from build123d import *

# Parameters (mm, degrees)
CYLINDER018_R               = 0.6
CYLINDER018_DEPTH           = 30
CYLINDER018_PLACEMENT_ANGLE = 45
ARRAY_COUNT                 = 6
CYLINDER014_R               = 0.4
CYLINDER014_DEPTH           = 2
CYLINDER012_R               = 0.41
CYLINDER012_DEPTH           = 0.8
CYLINDER013_R               = 0.7
CYLINDER013_DEPTH           = 0.55
FILLET003_R                 = 0.24
CYLINDER015_R               = 5
CYLINDER015_DEPTH           = 0.1
CYLINDER008_R               = 16
CYLINDER008_DEPTH           = 10
CYLINDER007_R               = 14
CYLINDER007_DEPTH           = 6.4
CYLINDER006_R               = 14
CYLINDER006_DEPTH           = 1
CYLINDER005_R               = 0.4
CYLINDER005_DEPTH           = 1
CYLINDER001_R               = 12.6
CYLINDER001_DEPTH           = 8
CYLINDER_R                  = 15
CYLINDER_DEPTH              = 8
CYLINDER002_R               = 15
CYLINDER002_DEPTH           = 1
FILLET_R                    = 0.7
FILLET001_R                 = 0.7
CHAMFER_SIZE                = 0.8


with BuildPart() as array:
    # Cylinder018 → Cylinder018 (new body)
    with BuildSketch(Plane.XY):
        Circle(CYLINDER018_R)
    extrude(amount=CYLINDER018_DEPTH)


with BuildPart() as array_1:
    # Cylinder018 placement: moved
    add(array.part.moved(Location((0, 0, -4.5))).rotate(Axis((0, 0, -4.5), (0, 1, 0)), CYLINDER018_PLACEMENT_ANGLE))

    # Array: Array ×6 about axis
    array_axis = Axis((0, 0, 0), (0, 0, 1))


with BuildPart() as array_2:
    add(array_1.part)
    for i in range(1, ARRAY_COUNT):
        add(array_1.part.rotate(array_axis, i * 360 / ARRAY_COUNT))


with BuildPart() as array_3:
    # Array placement: moved
    add(array_2.part.moved(Location((0, 0, -8.85))))


with BuildPart() as cylinder014:
    # Cylinder014 → Cylinder014 (new body)
    with BuildSketch(Plane.XY.offset(1)):
        Circle(CYLINDER014_R)
    extrude(amount=CYLINDER014_DEPTH)


with BuildPart() as cylinder012:
    # Cylinder012 → Cylinder012 (new body)
    with BuildSketch(Plane.XY.offset(1)):
        Circle(CYLINDER012_R)
    extrude(amount=CYLINDER012_DEPTH)


with BuildPart() as fillet003:
    # Cylinder013 → Cylinder013 (new body)
    with BuildSketch(Plane.XY.offset(1)):
        Circle(CYLINDER013_R)
    extrude(amount=CYLINDER013_DEPTH)

    # Fusion001: union Cylinder012
    add(cylinder012.part)

    # Fillet003
    fillet003_edges = [fillet003.edges().sort_by_distance(p)[0] for p in [
        (-0.41, 0, 1.55),
    ]]
    fillet(fillet003_edges, radius=FILLET003_R)


with BuildPart() as cut006:
    # Cylinder015 → Cylinder015 (new body)
    with BuildSketch(Plane.XY.offset(1)):
        Circle(CYLINDER015_R)
    extrude(amount=CYLINDER015_DEPTH)

    # Fusion002: union Fillet003
    add(fillet003.part)

    # Cut006: cut Cylinder014
    add(cylinder014.part, mode=Mode.SUBTRACT)


with BuildPart() as cylinder008:
    # Cylinder008 → Cylinder008 (new body)
    with BuildSketch(Plane.XY.offset(4)):
        Circle(CYLINDER008_R)
    extrude(amount=CYLINDER008_DEPTH)


with BuildPart() as cylinder007:
    # Cylinder007 → Cylinder007 (new body)
    with BuildSketch(Plane.XY.offset(1.6)):
        Circle(CYLINDER007_R)
    extrude(amount=CYLINDER007_DEPTH)


with BuildPart() as cylinder006:
    # Cylinder006 → Cylinder006 (new body)
    with BuildSketch(Plane.XY.offset(7)):
        Circle(CYLINDER006_R)
    extrude(amount=CYLINDER006_DEPTH)


with BuildPart() as cylinder005:
    # Cylinder005 → Cylinder005 (new body)
    with BuildSketch(Plane.XY):
        Circle(CYLINDER005_R)
    extrude(amount=CYLINDER005_DEPTH)


with BuildPart() as cylinder001:
    # Cylinder001 → Cylinder001 (new body)
    with BuildSketch(Plane.XY):
        Circle(CYLINDER001_R)
    extrude(amount=CYLINDER001_DEPTH)


with BuildPart() as cut:
    # Cylinder → Cylinder (new body)
    with BuildSketch(Plane.XY):
        Circle(CYLINDER_R)
    extrude(amount=CYLINDER_DEPTH)

    # Cut: cut Cylinder001
    add(cylinder001.part, mode=Mode.SUBTRACT)


with BuildPart() as cut009:
    # Cylinder002 → Cylinder002 (new body)
    with BuildSketch(Plane.XY):
        Circle(CYLINDER002_R)
    extrude(amount=CYLINDER002_DEPTH)

    # Fusion: union Cut
    add(cut.part)

    # Cut001: cut Cylinder005
    add(cylinder005.part, mode=Mode.SUBTRACT)

    # Cut003: cut Cylinder006
    add(cylinder006.part, mode=Mode.SUBTRACT)

    # Fillet
    fillet_edges = [cut009.edges().sort_by_distance(p)[0] for p in [
        (-15, 0, 8),
    ]]
    fillet(fillet_edges, radius=FILLET_R)

    # Fillet001
    fillet001_edges = [cut009.edges().sort_by_distance(p)[0] for p in [
        (-15, 0, 0),
    ]]
    fillet(fillet001_edges, radius=FILLET001_R)

    # Chamfer
    chamfer_edges = [cut009.edges().sort_by_distance(p)[0] for p in [
        (-0.4, 0, 0),
    ]]
    chamfer(chamfer_edges, length=CHAMFER_SIZE)

    # Cut007: cut Cylinder007
    add(cylinder007.part, mode=Mode.SUBTRACT)

    # Cut008: cut Cylinder008
    add(cylinder008.part, mode=Mode.SUBTRACT)

    # Fusion003: union Cut006
    add(cut006.part)

    # Cut009: cut Array
    add(array_3.part, mode=Mode.SUBTRACT)


solid = cut009.part
The listing builds one solid part. Answer for the finished solid, in the listing's coordinates (mm). A direction names the side the tool comes from. Coordinates: 2 decimals unless noted, no trailing zeros. Write each loop counter-clockwise with the first axis right and the second up, starting at its lowest first coordinate (ties: lowest second). Pieces come first, ordered by that corner, then holes. Notation, with made-up numbers: (46, 10.25) -> (51, 10.25) arc R28 cw to (51, 48.25) -> close; hole circle Ø2 at (9.5, 80). An arc over 180 degrees is marked (long way). One line per question, with ' | ' between items.
1. Section C-C (y = 0) is taken. State how many separate pieces and enclosed holes the cut face has, and give its area (3 significant figures).
Verdict:
separate pieces: 4 | enclosed holes: 0 | area: 31.6 mm^2
2. Which of the six approach directions +Z, -Z, +X, -X, +Y, -Y give full straight-line access (tool end or side, diameter ignored) to faces 4 (the cylindrical face through (-9.999, -7.667, 1.296)), 5 (the cylindrical face through (-13.7, 0, 1.2))?
Verdict:
face 4: +Z | face 5: none
3. Straight lines are drawn through the part: line 1 (Y direction, x = 0, z = 1.5); line 2 (X direction, y = 0, z = 1.25); line 3 (Z direction, x = -4, y = -1.5). For each, find the intervals that lie inside material, in ascending order.
Verdict:
line 1: y = -15 to -12.6, -0.7 to -0.4, 0.4 to 0.7, 12.6 to 15 | line 2: x = -13.75 to -12.6, -0.7 to -0.4, 0.4 to 0.7, 12.6 to 13.75 | line 3: z = 0 to 1.1
4. Section B-B (z = 3.6) is taken. Determine the outline of the cut face in (x, y), and give its area (3 significant figures).
Verdict:
outline: circle Ø30 at (0, 0); hole circle Ø28 at (0, 0) | area: 91.1 mm^2
5. Given pin 1 Ø1.5 at (x, z) = (-11, 3) entering from +Y; pin 2 Ø4 at (x, y) = (7.5, -9) entering from +Z; pin 3 Ø2 at (y, z) = (2.5, 1.5) entering from +X, each flat-ended and moving along its own axis, determine where each tip first touches the part or whether it passes through.
Verdict:
pin 1: stops at y = 10.95 | pin 2: stops at z = 1.6 | pin 3: stops at x = 14.92
6. For a pull along Y with two mould halves and no side action, classify faces 1 (the flat face through (3, 0, 0)), 2 (the flat face through (1, 0, 1.1)), 3 (the cylindrical face through (-14.985, 0.66, 2.327)) as released by +Y, released by -Y, zero draft, split by the parting line, or undercut.
Verdict:
face 1: zero draft | face 2: undercut | face 3: split by the parting line
